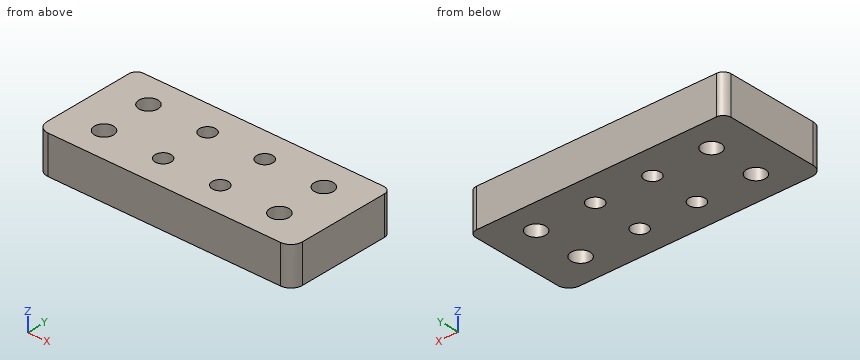
```python
from build123d import *

# Parameters (mm, degrees)
SKETCH_1_W                  = 67
SKETCH_1_H                  = 16
EXTRUDE_1_DEPTH             = 10
HOLE_WIZARD_M5_1_AT_2_COUNT = 2
HOLE_WIZARD_M5_1_AT_2_PITCH = 15
HOLE_WIZARD_M6_1_AT_2_COUNT = 2
HOLE_WIZARD_M6_1_AT_2_PITCH = 46
FILLET_1_R                  = 2
SKETCH_8_W                  = 67
SKETCH_8_H                  = 10
EXTRUDE_2_DEPTH             = 13
DELETE_START                = -33.5
DELETE_FACE_1_OUTLINE_W     = 27
DELETE_FACE_1_OUTLINE_H     = 10
DELETE_FACE_1_DEPTH         = 2.5
DELETE_START_2              = 31
DELETE_FACE_2_OUTLINE_W     = 27
DELETE_FACE_2_OUTLINE_H     = 10
DELETE_FACE_2_DEPTH         = 2.5
FILLET_2_R                  = 3


with BuildPart() as part:
    # 草图1 → 凸台-拉伸1 (new body)
    with BuildSketch(Plane.XY):
        Rectangle(SKETCH_1_W, SKETCH_1_H)
    extrude(amount=EXTRUDE_1_DEPTH)

    # 草图4 → M5 螺纹孔1 (revolve, cut)
    with BuildSketch(Plane(origin=(-7.5, 0, 10), x_dir=(0, -1, 0), z_dir=(1, 0, 0))):
        Polygon((0, 0), (0, 13.6618073), (2.1, 12.4), (2.1, 0), align=None)
    hole_wizard_m5_1 = revolve(axis=Axis((-7.5, 0, 16.35), (0, 0, -1)), mode=Mode.SUBTRACT)

    # M5 螺纹孔1 at 2: M5 螺纹孔1 ×2
    with Locations(*[(i * HOLE_WIZARD_M5_1_AT_2_PITCH, 0, 0) for i in range(1, HOLE_WIZARD_M5_1_AT_2_COUNT)]):
        add(hole_wizard_m5_1, mode=Mode.SUBTRACT)

    # 草图7 → M6 螺纹孔1 (revolve, cut)
    with BuildSketch(Plane(origin=(-23, 0, 10), x_dir=(0, -1, 0), z_dir=(1, 0, 0))):
        Polygon((0, 0), (0, 16.502151548), (2.5, 15), (2.5, 0), align=None)
    hole_wizard_m6_1 = revolve(axis=Axis((-23, 0, 16.35), (0, 0, -1)), mode=Mode.SUBTRACT)

    # M6 螺纹孔1 at 2: M6 螺纹孔1 ×2
    with Locations(*[(i * HOLE_WIZARD_M6_1_AT_2_PITCH, 0, 0) for i in range(1, HOLE_WIZARD_M6_1_AT_2_COUNT)]):
        add(hole_wizard_m6_1, mode=Mode.SUBTRACT)

    # 圆角1
    fillet_1_edges = [part.edges().sort_by_distance(p)[0] for p in [
        (33.5, -8, 5),
        (-33.5, -8, 5),
        (-33.5, 8, 5),
        (33.5, 8, 5),
    ]]
    fillet(fillet_1_edges, radius=FILLET_1_R)

    # 草图8 → 凸台-拉伸2 (add)
    with BuildSketch(Plane.XZ.offset(8)):
        with Locations((0, 5)):
            Rectangle(SKETCH_8_W, SKETCH_8_H)
    extrude(amount=EXTRUDE_2_DEPTH)

    # Delete Face 1: read off the stored shape, not the designer's step
    # Delete Face 1 outline → Delete Face 1 (add)
    with BuildSketch(Plane.YZ.offset(DELETE_START)):
        with Locations((-7.5, 5)):
            Rectangle(DELETE_FACE_1_OUTLINE_W, DELETE_FACE_1_OUTLINE_H)
    extrude(amount=DELETE_FACE_1_DEPTH)

    # Delete Face 2: read off the stored shape, not the designer's step
    # Delete Face 2 outline → Delete Face 2 (add)
    with BuildSketch(Plane.YZ.offset(DELETE_START_2)):
        with Locations((-7.5, 5)):
            Rectangle(DELETE_FACE_2_OUTLINE_W, DELETE_FACE_2_OUTLINE_H)
    extrude(amount=DELETE_FACE_2_DEPTH)

    # 镜向1: M5 螺纹孔1, M6 螺纹孔1 across plane
    add(hole_wizard_m5_1.mirror(Plane(origin=(0, -6.5, 0), x_dir=(0, 0, 1), z_dir=(0, -1, 0))), mode=Mode.SUBTRACT)
    add(hole_wizard_m6_1.mirror(Plane(origin=(0, -6.5, 0), x_dir=(0, 0, 1), z_dir=(0, -1, 0))), mode=Mode.SUBTRACT)

    # 镜向1 copy 1 sketch → 镜向1 copy 1 (revolve, cut)
    with BuildSketch(Plane(origin=(7.5, -13, 10), x_dir=(0, 1, 0), z_dir=(1, 0, 0))):
        Polygon((0, 0), (0, -13.6618073), (2.1, -12.4), (2.1, 0), align=None)
    revolve(axis=Axis((7.5, -13, 16.35), (0, 0, 1)), mode=Mode.SUBTRACT)

    # 镜向1 copy 2 sketch → 镜向1 copy 2 (revolve, cut)
    with BuildSketch(Plane(origin=(23, -13, 10), x_dir=(0, 1, 0), z_dir=(1, 0, 0))):
        Polygon((0, 0), (0, -16.502151548), (2.5, -15), (2.5, 0), align=None)
    revolve(axis=Axis((23, -13, 16.35), (0, 0, 1)), mode=Mode.SUBTRACT)

    # 圆角2
    fillet_2_edges = [part.edges().sort_by_distance(p)[0] for p in [
        (-33.5, -21, 5),
        (33.5, -21, 5),
    ]]
    fillet(fillet_2_edges, radius=FILLET_2_R)


solid = part.part
```
Source: CAD feature listing. Evaluate the final solid. Frame: model axes, mm. Round coordinates to 2 decimals unless told otherwise and drop trailing zeros. Loops run counter-clockwise (first coordinate to the right, second up) from the corner with the lowest first, then second, coordinate; pieces in that order, holes last. Notation, with made-up numbers: M -3,-16 L 40,-16 A10 ccw 40,-10 Z; hole C 70,45 d5. An arc over 180 degrees is marked long. Use a Markdown table: item, result. Add a question column.
1. Cut plane C-C, the plane z = 7.5. State how many separate pieces and enclosed holes the cut face has, and give its area (3 significant figures).
2. Cut plane A-A, the plane x = -7.5. Output: boundary loops of the cut face in (y, z), and give its area (3 significant figures).
3. Cut plane D-D, the plane x = -23. Output: boundary loops of the cut face in (y, z).
4. Cut plane B-B, the plane y = -13. Output: boundary loops of the cut face in (x, z), and give its area (3 significant figures).
5. Contact query for a flat-ended pin moving along its axis: pin 1 (3 mm diameter, centred on x = -23, y = -13, fed in from +Z). Output: stop coordinate, or through.
6. Ray query, line 1 along X through (y, z) = (0, 7.25); line 2 along Y through (x, z) = (7.5, 4.25); line 3 along Y through (x, z) = (23, 7.25). Return the intervals inside material, ascending. Write a range as [from, to].
Solution:
| question | item | result |
|---|---|---|
| 1 | separate pieces | 1 |
| 1 | enclosed holes | 8 |
| 1 | area | 1,800 mm2 |
| 2 | outline | M -21,0 L -15.1,0 L -15.1,10 L -21,10 Z; M -10.9,0 L -2.1,0 L -2.1,10 L -10.9,10 Z; M 2.1,0 L 8,0 L 8,10 L 2.1,10 Z |
| 2 | area | 206 mm2 |
| 3 | outline | M -21,0 L -15.5,0 L -15.5,10 L -21,10 Z; M -10.5,0 L -2.5,0 L -2.5,10 L -10.5,10 Z; M 2.5,0 L 8,0 L 8,10 L 2.5,10 Z |
| 4 | outline | M -33.5,0 L -25.5,0 L -25.5,10 L -33.5,10 Z; M -20.5,0 L -9.6,0 L -9.6,10 L -20.5,10 Z; M -5.4,0 L 5.4,0 L 5.4,10 L -5.4,10 Z; M 9.6,0 L 20.5,0 L 20.5,10 L 9.6,10 Z; M 25.5,0 L 33.5,0 L 33.5,10 L 25.5,10 Z |
| 4 | area | 486 mm2 |
| 5 | pin 1 | passes through |
| 6 | line 1 | x = [-33.5, -25.5], [-20.5, -9.6], [-5.4, 5.4], [9.6, 20.5], [25.5, 33.5] |
| 6 | line 2 | y = [-21, -15.1], [-10.9, -2.1], [2.1, 8] |
| 6 | line 3 | y = [-21, -15.5], [-10.5, -2.5], [2.5, 8] |
